Can you work these out from the model? Positions are in its coordinate system, mm. Face numbers are marked on the shaded views. A direction names the side the tool comes from. Round coordinates to 2 decimals unless told otherwise and drop trailing zeros. Order: outer loops, then holes, each group sorted by start corner. A loop starts at its lowest first (then second) coordinate and runs counter-clockwise, first axis right, second up. Notation, with made-up numbers: M -12.5,29.5 L 27.5,29.5 A24 ccw 27.5,62.5 Z; hole C -40,25.25 d2. An arc over 180 degrees is marked long. Answer as a JSON object with one key per item and string values. Group by question number.
```python
from build123d import *

# Parameters (mm, degrees)
SKETCH1_W                 = 200
SKETCH1_H                 = 120
BOSS_EXTRUDE1_DEPTH       = 40
CUT_EXTRUDE2_DEPTH        = 40
CUT_EXTRUDE3_DEPTH        = 40
CUT_EXTRUDE4_DEPTH        = 40
SKETCH5_W                 = 208.7299617
SKETCH5_H                 = 60
CUT_EXTRUDE5_DEPTH        = 10
CUT_EXTRUDE6_DEPTH        = 116
BOSS_EXTRUDE2_DEPTH       = 20
CUT_EXTRUDE7_DEPTH        = 10
SKETCH9_R                 = 10
BOSS_EXTRUDE3_DEPTH       = 30
SKETCH10_R                = 10
CUT_EXTRUDE8_DEPTH        = 69
SKETCH11_R                = 20
SKETCH11_R_2              = 10
BOSS_EXTRUDE4_DEPTH       = 20
SKETCH12_R                = 35
SKETCH12_R_2              = 20
CUT_EXTRUDE9_DEPTH        = 10
BOSS_EXTRUDE10_DEPTH      = 10
BOSS_EXTRUDE10_DEPTH_BACK = 36
BOSS_EXTRUDE11_DEPTH      = 20
CUT_EXTRUDE10_DEPTH       = 20
SKETCH17_W                = 10
SKETCH17_H                = 10
CUT_EXTRUDE11_DEPTH       = 20
SKETCH18_W                = 181.961524227
SKETCH18_H                = 60
CUT_EXTRUDE12_DEPTH       = 20


with BuildPart() as part:
    # Sketch1 → Boss-Extrude1 (new body)
    with BuildSketch(Plane(origin=(0, 0, 0), x_dir=(1, 0, 0), z_dir=(0, 1, 0))):
        with Locations((100, 60)):
            Rectangle(SKETCH1_W, SKETCH1_H)
    extrude(amount=BOSS_EXTRUDE1_DEPTH)

    # Sketch2 → Cut-Extrude2 (cut)
    with BuildSketch(Plane(origin=(0, 40, 0), x_dir=(1, 0, 0), z_dir=(0, 1, 0))):
        Polygon((0, 110), (50, 110), (90, 110), (90, 120), (0, 120), align=None)
        with BuildLine():
            ThreePointArc((0, 60), (14.644660941, 95.355339059), (50, 110))
            Line((50, 110), (0, 110))
            Line((0, 110), (0, 60))
        make_face()
        with BuildLine():
            ThreePointArc((50, 10), (14.644660941, 24.644660941), (0, 60))
            Line((0, 60), (0, 0))
            Line((0, 0), (90, 0))
            Line((90, 0), (90, 10))
            Line((90, 10), (50, 10))
        make_face()
    extrude(amount=-CUT_EXTRUDE2_DEPTH, mode=Mode.SUBTRACT)

    # Sketch3 → Cut-Extrude3 (cut)
    with BuildSketch(Plane(origin=(0, 40, 0), x_dir=(1, 0, 0), z_dir=(0, 1, 0))):
        with BuildLine():
            Line((90, 110), (90, 120))
            Line((90, 120), (100, 120))
            ThreePointArc((100, 120), (97.071067812, 112.928932188), (90, 110))
        make_face()
    extrude(amount=-CUT_EXTRUDE3_DEPTH, mode=Mode.SUBTRACT)

    # Sketch4 → Cut-Extrude4 (cut)
    with BuildSketch(Plane(origin=(0, 40, 0), x_dir=(1, 0, 0), z_dir=(0, 1, 0))):
        with BuildLine():
            Line((90, 10), (90, 0))
            Line((90, 0), (100, 0))
            ThreePointArc((100, 0), (97.071067812, 7.071067812), (90, 10))
        make_face()
    extrude(amount=-CUT_EXTRUDE4_DEPTH, mode=Mode.SUBTRACT)

    # Sketch5 → Cut-Extrude5 (cut)
    with BuildSketch(Plane.XZ):
        with Locations((95.63501915, -60)):
            Rectangle(SKETCH5_W, SKETCH5_H)
    extrude(amount=-CUT_EXTRUDE5_DEPTH, mode=Mode.SUBTRACT)

    # Sketch6 → Cut-Extrude6 (cut)
    with BuildSketch(Plane(origin=(0, 40, 0), x_dir=(1, 0, 0), z_dir=(0, 1, 0))):
        with BuildLine():
            Line((200, 120), (140, 120))
            ThreePointArc((140, 120), (182.426406871, 102.426406871), (200, 60))
            Line((200, 60), (200, 120))
        make_face()
        with BuildLine():
            Line((200, 0), (200, 60))
            ThreePointArc((200, 60), (182.426406871, 17.573593129), (140, 0))
            Line((140, 0), (200, 0))
        make_face()
    extrude(amount=-CUT_EXTRUDE6_DEPTH, mode=Mode.SUBTRACT)

    # Sketch7 → Boss-Extrude2 (add)
    with BuildSketch(Plane(origin=(0, 40, 0), x_dir=(1, 0, 0), z_dir=(0, 1, 0))):
        with BuildLine():
            Line((140, 110), (140, 120))
            ThreePointArc((140, 120), (200, 60), (140, 0))
            Line((140, 0), (140, 10))
            ThreePointArc((140, 10), (190, 60), (140, 110))
        make_face()
    extrude(amount=BOSS_EXTRUDE2_DEPTH)

    # Sketch8 → Cut-Extrude7 (cut)
    with BuildSketch(Plane(origin=(0, 40, 0), x_dir=(1, 0, 0), z_dir=(0, 1, 0))):
        with BuildLine():
            Line((50, 90), (10, 90))
            ThreePointArc((10, 90), (0, 60), (10, 30))
            Line((10, 30), (50, 30))
            ThreePointArc((50, 30), (80, 60), (50, 90))
        make_face()
    extrude(amount=-CUT_EXTRUDE7_DEPTH, mode=Mode.SUBTRACT)

    # Sketch9 → Boss-Extrude3 (add)
    with BuildSketch(Plane(origin=(0, 30, 0), x_dir=(1, 0, 0), z_dir=(0, 1, 0))):
        with Locations((50, 60)):
            Circle(SKETCH9_R)
    extrude(amount=BOSS_EXTRUDE3_DEPTH)

    # Sketch10 → Cut-Extrude8 (cut)
    with BuildSketch(Plane(origin=(0, 40, 0), x_dir=(1, 0, 0), z_dir=(0, 1, 0))):
        with Locations((140, 60)):
            Circle(SKETCH10_R)
    extrude(amount=-CUT_EXTRUDE8_DEPTH, mode=Mode.SUBTRACT)

    # Sketch11 → Boss-Extrude4 (add)
    with BuildSketch(Plane(origin=(0, 40, 0), x_dir=(1, 0, 0), z_dir=(0, 1, 0))):
        with Locations((140, 60)):
            Circle(SKETCH11_R)
        with Locations((140, 60)):
            Circle(SKETCH11_R_2, mode=Mode.SUBTRACT)
    extrude(amount=BOSS_EXTRUDE4_DEPTH)

    # Sketch12 → Cut-Extrude9 (cut)
    with BuildSketch(Plane(origin=(0, 40, 0), x_dir=(1, 0, 0), z_dir=(0, 1, 0))):
        with Locations((140, 60)):
            Circle(SKETCH12_R)
        with Locations((140, 60)):
            Circle(SKETCH12_R_2, mode=Mode.SUBTRACT)
    extrude(amount=-CUT_EXTRUDE9_DEPTH, mode=Mode.SUBTRACT)

    # Sketch14 → Boss-Extrude10 (add, two sides)
    with BuildSketch(Plane(origin=(0, 40, 0), x_dir=(1, 0, 0), z_dir=(0, 1, 0))) as boss_extrude10_sk:
        with BuildLine():
            Line((174.641016151, 65), (160, 65))
            Line((160, 65), (160, 55))
            Line((160, 55), (174.641016151, 55))
            ThreePointArc((174.641016151, 55), (174.91013868, 57.493564812), (175, 60))
            ThreePointArc((175, 60), (174.91013868, 62.506435188), (174.641016151, 65))
        make_face()
        with BuildLine():
            Line((158.948525297, 65), (160, 65))
            Line((160, 65), (160, 55))
            Line((160, 55), (158.948525297, 55))
            ThreePointArc((158.948525297, 55), (159.597107209, 60), (158.948525297, 65))
        make_face()
        with BuildLine():
            Line((189.749371855, 65), (174.641016151, 65))
            ThreePointArc((174.641016151, 65), (174.91013868, 62.506435188), (175, 60))
            ThreePointArc((175, 60), (174.91013868, 57.493564812), (174.641016151, 55))
            Line((174.641016151, 55), (189.749371855, 55))
            ThreePointArc((189.749371855, 55), (190, 60), (189.749371855, 65))
        make_face()
    extrude(amount=BOSS_EXTRUDE10_DEPTH)
    extrude(boss_extrude10_sk.sketch, amount=-BOSS_EXTRUDE10_DEPTH_BACK)

    # Sketch15 → Boss-Extrude11 (add)
    with BuildSketch(Plane(origin=(0, 30, 0), x_dir=(1, 0, 0), z_dir=(0, 1, 0))):
        with BuildLine():
            Line((120.635083269, 55), (120.635083269, 65))
            ThreePointArc((120.635083269, 65), (120, 60), (120.635083269, 55))
        make_face()
        with BuildLine():
            ThreePointArc((120.635083269, 55), (120, 60), (120.635083269, 65))
            Line((120.635083269, 65), (105.358983849, 65))
            ThreePointArc((105.358983849, 65), (105, 60), (105.358983849, 55))
            Line((105.358983849, 55), (120.635083269, 55))
        make_face()
    extrude(amount=BOSS_EXTRUDE11_DEPTH)

    # Sketch16 → Cut-Extrude10 (cut)
    with BuildSketch(Plane.XY.offset(-55)):
        Polygon((120.635083269, 50), (105.358983849, 40), (105.358983849, 50), align=None)
    extrude(amount=-CUT_EXTRUDE10_DEPTH, mode=Mode.SUBTRACT)

    # Sketch17 → Cut-Extrude11 (cut)
    with BuildSketch(Plane(origin=(105.358983849, 0, 0), x_dir=(0, 0, -1), z_dir=(1, 0, 0))):
        with Locations((60, 45)):
            Rectangle(SKETCH17_W, SKETCH17_H)
    extrude(amount=-CUT_EXTRUDE11_DEPTH, mode=Mode.SUBTRACT)

    # Sketch18 → Cut-Extrude12 (cut)
    with BuildSketch(Plane.XZ.offset(-10)):
        with Locations((100.980762114, -60)):
            Rectangle(SKETCH18_W, SKETCH18_H)
    extrude(amount=CUT_EXTRUDE12_DEPTH, mode=Mode.SUBTRACT)


solid = part.part
```
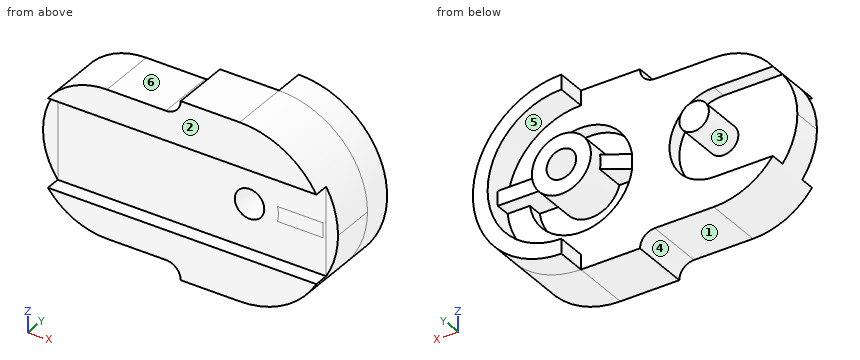
1) If we section it at D-D on x = 187: Write out the boundary of the cut face in (y, z), plus the area to 3 significant figures.
2) We'd pull the mould along X, two halves only. Please class the marked faces 4, 5 and 6: +X half, -X half, draft (parallel to the pull), parting line (faces both ways), or undercut.
3) I need wall thicknesses on line 1 along X through (y, z) = (31.25, -60); line 2 along X through (y, z) = (24.75, -60); line 3 along Z through (x, y) = (140, 26). Which ranges of each line are inside material? Lowest first, please.
4) For pin 1 (3 mm diameter, centred on y = 54.5, z = -116, fed in from -X); pin 2 (8 mm diameter, centred on x = 78, y = 5.5, fed in from +Z); pin 3 (18 mm diameter, centred on x = 140, z = -60, fed in from +Y); pin 4 (0.7 mm diameter, centred on x = 120, z = -61, fed in from -Y), each with a flat end and sliding along its axis, tell me the tip position at first contact or that it passes through.
5) If we section it at C-C on z = -33: Write out the boundary of the cut face in (x, y), plus the area to 3 significant figures.
6) If we section it at B-B on x = 134.5: Write out the boundary of the cut face in (y, z), plus the area to 3 significant figures.
7) Which directions (+Z, -Z, +X, -X, +Y, -Y) give clear straight access to the entire face, cutting with the end or side of a thin tool? Please do the marked faces 1, 2 and 3.
8) If we section it at A-A on y = 55.5: Write out the boundary of the cut face in (x, z), plus the area to 3 significant figures.
Findings:
{
 "1": {"outline": "M 0,-97.3 L 60,-97.3 L 60,-77.06 L 40,-77.06 L 40,-65 L 50,-65 L 50,-55 L 40,-55 L 40,-42.94 L 60,-42.94 L 60,-22.7 L 0,-22.7 L 0,-30 L 10,-30 L 10,-90 L 0,-90 Z", "area": "3,290 mm^2"},
 "2": {"face 4": "-X half", "face 5": "undercut", "face 6": "draft"},
 "3": {"line 1": "x = 40 to 60, 80 to 130, 150 to 200", "line 2": "x = 0 to 130, 150 to 200", "line 3": "z = -120 to -70, -50 to 0"},
 "4": {"pin 1": "stops at x = 140", "pin 2": "stops at z = -10", "pin 3": "passes through", "pin 4": "stops at y = 10"},
 "5": {"outline": "M 7.92,10 L 193.58,10 L 193.58,60 L 182.08,60 L 182.08,40 L 162.27,40 L 162.27,30 L 117.73,30 L 117.73,40 L 63.08,40 L 63.08,30 L 7.92,30 Z", "area": "4,800 mm^2"},
 "6": {"outline": "M 0,-120 L 40,-120 L 40,-94.57 L 30,-94.57 L 30,-79.23 L 60,-79.23 L 60,-68.35 L 10,-68.35 L 10,-90 L 0,-90 Z; M 0,-30 L 10,-30 L 10,-51.65 L 60,-51.65 L 60,-40.77 L 30,-40.77 L 30,-25.43 L 40,-25.43 L 40,0 L 0,0 Z", "area": "3,830 mm^2"},
 "7": {"face 1": "-Z, -X, +Y, -Y", "face 2": "+Z, -Z, +X, -X, -Y", "face 3": "+Y"},
 "8": {"outline": "C 50,-60 d20; C 140,-60 d40; M 140,-120 A60 ccw 140,0 L 140,-10 A50 cw 140,-110 Z; hole C 140,-60 d20", "area": "2,980 mm^2"}
}
